Model file for the job. Use its own axes, mm. Face numbers are marked on the shaded views. Coordinates: 2 decimals unless noted, no trailing zeros. Order: outer loops, then holes, each group sorted by start corner. A loop starts at its lowest first (then second) coordinate and runs counter-clockwise, first axis right, second up. Notation, with made-up numbers: (79, 44.25) -> (131, 44.25) arc R10 cw to (131, 63.25) -> close; hole circle Ø11 at (55.25, 36). An arc over 180 degrees is marked (long way). Use CSV: the item, a comma, the result in double quotes. Start each with the question number.
(1) Cut at C-C on y = 5. Write the cut outline in (x, z).
(2) Pull direction X, two halves, no side cores. Call the marked faces 1 and 2: pulls with the +X half, pulls with the -X half, needs draft (parallel to the pull), parting line crosses it, or undercut.
(3) Cut at D-D on x = 14. Write the cut outline in (y, z), plus the area to 3 significant figures.
(4) Cut at A-A on z = 2.5. Write the cut outline in (x, y).
(5) Probe L1, parallel to X at y = 3.8, z = 3.7; L2, parallel to X at y = 3.25, z = 2.3; L3, parallel to Y at x = 7, z = 1.3. List the from-to ranges inside material, lowest first.
(6) Pin check, flat tips, straight feed: pin 1 Ø1 at (x, y) = (33.5, 5.5) entering from -Z; pin 2 Ø1.6 at (x, z) = (49.5, 2) entering from -Y; pin 3 Ø0.6 at (x, y) = (30, 4.5) entering from +Z; pin 4 Ø1.5 at (x, y) = (31.5, 3) entering from -Z. Stop position of each tip, or through.
(7) Cut at B-B on x = 50. Write the cut outline in (y, z).
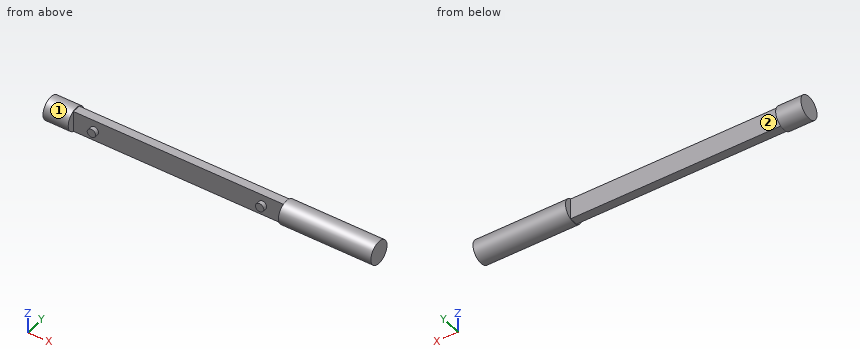
Autodesk Inventor part; units mm, degrees
ref_plane "YZ Plane" through (0, 0, 0) normal (1, 0, 0) x (0, 1, 0)
ref_plane "XZ Plane" through (0, 0, 0) normal (0, 1, 0) x (-1, 0, 0)
ref_plane "XY Plane" through (0, 0, 0) normal (0, 0, 1) x (1, 0, 0)
sketch "Esquisse1" plane through (0, 0, 0) normal (0, 0, 1) x (1, 0, 0)
  line L0 (0, 10) -> (5, 10)
  line L1 (5, 6) -> (5, 10)
  line L2 (5, 6) -> (55, 6)
  line L3 (55, 6) -> (55, 10)
  line L4 (55, 0) -> (55, 4)
  line L5 (55, 4) -> (5, 4)
  line L6 (5, 6) -> (5, 4)
  line L7 (55, 6) -> (55, 4)
  point P0 (0, 0)
  point P1 (25, 10)
  dimension "d39" = 50
  dimension "d40" = 5
extrude "Extrusion1" add sketch "Esquisse1" along normal blind 5
sketch "Esquisse9" plane through (5, 6, 0) normal (0, 1, 0) x (1, 0, 0)
  line L0 (0, 0) -> (5, 0)
  line L1 (5, 0) -> (45, 0)
  line L2 (0, 0) -> (50, 0)
  line L3 (45, 0) -> (45, -2.5)
  line L4 (5, 0) -> (5, -2.5)
  circle A0 centre (5, -2.5) radius 1
  circle A1 centre (45, -2.5) radius 1
  point P0 (-5, 0)
  dimension "d42" = 5
  dimension "d43" = 40
  dimension "d44" = 2
  dimension "d45" = 2
extrude "Extrusion9" add sketch "Esquisse9" against normal blind 3
sketch "Esquisse10" plane through (55, 4, 0) normal (1, 0, 0) x (0, 0, -1)
  line L0 (0, 0) -> (0, 2)
  line L1 (0, 1) -> (-5, 1)
  line L2 (-5, 0) -> (-5, 2)
  circle A0 centre (-2.5, 1) radius 2.75
  point P0 (0, -4)
  dimension "d50" = 5.5
extrude "Extrusion10" add sketch "Esquisse10" along normal blind 22
sketch "Esquisse11" plane through (5, 4, 0) normal (-1, 0, 0) x (0, 0, 1)
  circle A0 centre (2.5, 1) radius 2.75
  circle A1 centre (2.5, 1) radius 2.75
  point P0 (0, -4)
extrude "Extrusion11" add sketch "Esquisse11" along normal blind 6
properties part number "Cheville"
Outcome:
1,outline,"(-1, -0.25) -> (5, -0.25) -> (5, 0) -> (55, 0) -> (55, -0.25) -> (77, -0.25) -> (77, 5.25) -> (55, 5.25) -> (55, 5) -> (5, 5) -> (5, 5.25) -> (-1, 5.25) -> close"
2,face 1,"needs draft"
2,face 2,"undercut"
3,outline,"(4, 0) -> (6, 0) -> (6, 5) -> (4, 5) -> close"
3,area,"10.0 mm2"
4,outline,"(-1, 2.25) -> (5, 2.25) -> (5, 4) -> (9, 4) -> (9, 3) -> (11, 3) -> (11, 4) -> (49, 4) -> (49, 3) -> (51, 3) -> (51, 4) -> (55, 4) -> (55, 2.25) -> (77, 2.25) -> (77, 7.75) -> (55, 7.75) -> (55, 6) -> (5, 6) -> (5, 7.75) -> (-1, 7.75) -> close"
5,L1,"-1 to 5, 55 to 77"
5,L2,"-1 to 5, 9.02 to 10.98, 49.02 to 50.98, 55 to 77"
5,L3,"4 to 6"
6,pin 1,"z = 0"
6,pin 2,"y = 3"
6,pin 3,"z = 5"
6,pin 4,"through"
7,outline,"(3, 1.5) -> (4, 1.5) -> (4, 0) -> (6, 0) -> (6, 5) -> (4, 5) -> (4, 3.5) -> (3, 3.5) -> close"
